from build123d import *

# Parameters (mm, degrees)
F0_W     = 50
F0_H     = 1.5
F1_DEPTH = 25
F3_W     = 0.5
F3_H     = 25
F3_W_2   = 0.8
F3_W_3   = 1
F3_W_4   = 1.4
F3_W_5   = 1.2
F3_W_6   = 1.6
F3_W_7   = 2
F3_W_8   = 2.5
F3_W_9   = 3
F4_DEPTH = 10


with BuildPart() as f1:
    # F0 (on Front) → F1 (new body)
    with BuildSketch(Plane.XZ):
        with Locations((25, 0.75)):
            Rectangle(F0_W, F0_H)
    extrude(amount=-F1_DEPTH)

    # F3 (on offset) → F4 (join)
    with BuildSketch(Plane.XY.offset(1.5)):
        with Locations((2.25, 12.5)):
            Rectangle(F3_W, F3_H)
        with Locations((6.9, 12.5)):
            Rectangle(F3_W_2, F3_H)
        with Locations((11.8, 12.5)):
            Rectangle(F3_W_3, F3_H)
        with Locations((24.3, 12.5)):
            Rectangle(F3_W_4, F3_H)
        with Locations((16.9, 12.5)):
            Rectangle(F3_W_5, F3_H)
        with Locations((29.8, 12.5)):
            Rectangle(F3_W_6, F3_H)
        with Locations((35.6, 12.5)):
            Rectangle(F3_W_7, F3_H)
        with Locations((41.85, 12.5)):
            Rectangle(F3_W_8, F3_H)
        with Locations((47.6, 12.5)):
            Rectangle(F3_W_9, F3_H)
    extrude(amount=F4_DEPTH)


solid = f1.part
CAD build for the part. Positions are in the model's coordinates, mm. A direction names the side the tool comes from. Give positions to 0.01 mm unless a question says otherwise; leave off trailing zeros. Loops run counter-clockwise (first coordinate to the right, second up) from the corner with the lowest first, then second, coordinate; pieces in that order, holes last. Notation, with made-up numbers: M 46,30.25 L 55,30.25 A17 cw 55,37.25 Z; hole C 74.25,67.5 d9. An arc over 180 degrees is marked long. Answer in a Markdown table with one row per item. Add a question column.
Item 1: Tool access for faces 1 (the face through (30, 0, 6)), 2 (the face through (17, 13, 11.5)), 3 (the face through (1, 12, 1.5)), 4 (the face through (39, 12, 1.5)), 5 (the face through (49.1, 12, 6)): list every direction of +Z, -Z, +X, -X, +Y, -Y with a clear straight run to the whole face (end or side of a thin tool).
Item 2: Drop flat-ended pins along their axis: P1, Ø5, axis at y = 11, z = 7, coming from the +X side; P2, Ø1.5, axis at x = 39.5, y = 14.5, coming from the -Z side; P3, Ø1, axis at x = 10, y = 17, coming from the +Z side; P4, Ø3, axis at y = 6.5, z = 6, coming from the -X side. Give the stop position or say it passes through.
Item 3: Probe probe 1 along Z at (x, y) = (38, 22.5). List the from-to ranges inside material, lowest first.
Item 4: Mould opens along X. For faces 6 (the face through (2, 12, 6)), 7 (the face through (12, 13, 11.5)), 8 (the face through (33, 12, 1.5)) say: +X half, -X half, draft (parallel to the pull), parting line (faces both ways), or undercut.
Item 5: Band-saw the part on A-A on z = 6.5. Give the number of separate pieces and of enclosed holes in the cut face, then the cut area to 3 significant figures.
Item 6: Band-saw the part on B-B on x = 6. Give the cut face in (y, z), then the cut area to 3 significant figures.
Reply:
| question | item | result |
|---|---|---|
| 1 | face 1 | +Z, -Z, +X, -X, -Y |
| 1 | face 2 | +Z, +X, -X, +Y, -Y |
| 1 | face 3 | +Z, -X, +Y, -Y |
| 1 | face 4 | +Z, +Y, -Y |
| 1 | face 5 | +Z, +X, +Y, -Y |
| 2 | P1 | stops at x = 49.1 |
| 2 | P2 | stops at z = 0 |
| 2 | P3 | stops at z = 1.5 |
| 2 | P4 | stops at x = 2 |
| 3 | probe 1 | z = 0 to 1.5 |
| 4 | face 6 | -X half |
| 4 | face 7 | draft |
| 4 | face 8 | undercut |
| 5 | separate pieces | 9 |
| 5 | enclosed holes | 0 |
| 5 | area | 350 mm^2 |
| 6 | outline | M 0,0 L 25,0 L 25,1.5 L 0,1.5 Z |
| 6 | area | 37.5 mm^2 |
